```python
from build123d import *

# Parameters (mm, degrees)
F0_R     = 10.16
F1_DEPTH = 15.7734
F2_DEPTH = 40.2336
F3_R     = 3.302


with BuildPart() as f1:
    # F0 (on Top) → F1 (new body)
    with BuildSketch(Plane.XY):
        with BuildLine():
            ThreePointArc((9.512184, 26.945296), (23.327466, 16.503332), (28.575, 0))
            ThreePointArc((28.575, 0), (23.327466, -16.503332), (9.512184, -26.945296))
            Line((9.512184, -26.945296), (57.191927, -18.776418))
            ThreePointArc((57.191927, -18.776418), (73.025, 0), (57.191927, 18.776418))
            Line((57.191927, 18.776418), (9.512184, 26.945296))
        make_face()
        with Locations((53.975, 0)):
            Circle(F0_R, mode=Mode.SUBTRACT)
    extrude(amount=F1_DEPTH)

    # F0 (on Top) → F2 (join)
    with BuildSketch(Plane.XY):
        with BuildLine():
            ThreePointArc((9.512184, -26.945296), (23.327466, -16.503332), (28.575, 0))
            ThreePointArc((28.575, 0), (23.327466, 16.503332), (9.512184, 26.945296))
            ThreePointArc((9.512184, 26.945296), (-28.575, 0), (9.512184, -26.945296))
        make_face()
        with BuildLine():
            ThreePointArc((13.447765, -4.826), (-14.2875, 0), (13.447765, 4.826))
            Line((13.447765, 4.826), (16.4084, 4.826))
            Line((16.4084, 4.826), (16.4084, -4.826))
            Line((16.4084, -4.826), (13.447765, -4.826))
        make_face(mode=Mode.SUBTRACT)
    extrude(amount=F2_DEPTH)

    # F3
    f3_edges = [f1.edges().sort_by_distance(p)[0] for p in [
        (-9.512184, 26.945296, 40.2336),
    ]]
    fillet(f3_edges, radius=F3_R)


solid = f1.part
```
Source: CAD feature listing. Evaluate the final solid. Frame: model axes, mm. A direction names the side the tool comes from. Give positions to 0.01 mm unless a question says otherwise; leave off trailing zeros. Order: outer loops, then holes, each group sorted by start corner. A loop starts at its lowest first (then second) coordinate and runs counter-clockwise, first axis right, second up. Notation, with made-up numbers: (3, -34.75) -> (50, -34.75) arc R18 cw to (50, -8.75) -> close; hole circle Ø7 at (41.5, 82). An arc over 180 degrees is marked (long way). Use a Markdown table: item, result.
Q1. First-contact query: P1, Ø12, axis at x = 35.5, y = 13.5, coming from the +Z side; P2, Ø6, axis at x = 28.5, z = 25.5, coming from the +Y side (3 decimals); P3, Ø1.5, axis at x = 15, z = 13.5, coming from the +Y side; P4, Ø1, axis at x = 57, y = -20, coming from the +Z side. Flat tips, straight axial feed; report the tip coordinate or a pass-through.
A:
| item | result |
|---|---|
| P1 | z = 15.77 |
| P2 | y = 12.895 |
| P3 | y = 26.13 |
| P4 | through |
Q2. Access query for faces 5 (the face through (16.408, 0, 20)), 6 (the face through (11, -11, 40.234)). Directions: +Z, -Z, +X, -X, +Y, -Y. A direction counts if a zero-diameter tool reaches every point of the face in a straight line with its end or side. Return the directions, or none.
A:
| item | result |
|---|---|
| face 5 | +Z, -Z |
| face 6 | +Z, +X, -X, +Y, -Y |
Q3. Section B-B (x = 63). Return the cut outline in (y, z).
A:
| item | result |
|---|---|
| outline | (-16.78, 0) -> (-4.67, 0) -> (-4.67, 15.77) -> (-16.78, 15.77) -> close; (4.67, 0) -> (16.78, 0) -> (16.78, 15.77) -> (4.67, 15.77) -> close |
Q4. Material intervals for line 1 (Y direction, x = 0, z = 16) (1 decimal); line 2 (Y direction, x = -8, z = 35); line 3 (Z direction, x = 57.5, y = 17), sorted ascending. Write a range as [from, to].
A:
| item | result |
|---|---|
| line 1 | [-28.6, -14.3], [14.3, 28.6] |
| line 2 | [-27.43, -11.84], [11.84, 27.43] |
| line 3 | [0, 15.77] |
Q5. Pull-direction query (Y, two-part tool) for faces 1 (the face through (15, -4.826, 20)), 2 (the face through (73.02, -0.37, 7.78)), 3 (the face through (33.7, 22.8, 7.8)), 4 (the face through (41, 0, 15.773)); classes: +Y half, -Y half, draft (parallel to the pull), parting line (faces both ways), or undercut.
A:
| item | result |
|---|---|
| face 1 | undercut |
| face 2 | parting line |
| face 3 | +Y half |
| face 4 | draft |
Q6. Section C-C (z = 9.5). State how many separate pieces and enclosed holes the cut face has, and give its area (3 significant figures).
A:
| item | result |
|---|---|
| separate pieces | 1 |
| enclosed holes | 2 |
| area | 3,460 mm^2 |
